```python
from build123d import *

# Parameters (mm, degrees)
SKETCH007_W     = 120
SKETCH007_H     = 120
PAD002_DEPTH    = 100
POCKET005_DEPTH = 100.001
SKETCH009_R     = 1.9
POCKET006_DEPTH = 16
SKETCH010_W     = 3.9
SKETCH010_H     = 62
POCKET007_DEPTH = 114
SKETCH011_R     = 1.9
POCKET008_DEPTH = 16
SKETCH012_R     = 1.9
POCKET009_DEPTH = 120.001
SKETCH013_W     = 106
SKETCH013_H     = 50
POCKET010_DEPTH = 3
SKETCH014_R     = 3
POCKET011_DEPTH = 120.001
SKETCH015_W     = 10
SKETCH015_H     = 10
POCKET012_DEPTH = 3


with BuildPart() as part:
    # Sketch007 → Pad002 (new body)
    with BuildSketch(Plane.XY):
        with Locations((75, 75)):
            Rectangle(SKETCH007_W, SKETCH007_H)
    extrude(amount=PAD002_DEPTH)

    # Sketch008 (on Face5 of Pad002) → Pocket005 (cut, through all)
    with BuildSketch(Plane(origin=(0, 0, 0), x_dir=(1, 0, 0), z_dir=(0, 0, -1))):
        with BuildLine():
            Line((21.9, -18), (128.1, -18))
            Line((128.1, -18), (128.1, -18.9))
            ThreePointArc((128.1, -18.9), (128.97868, -21.02132), (131.1, -21.9))
            Line((132, -21.9), (131.1, -21.9))
            Line((132, -21.9), (132, -128.1))
            Line((132, -128.1), (131.1, -128.1))
            ThreePointArc((131.1, -128.1), (128.97868, -128.97868), (128.1, -131.1))
            Line((128.1, -132), (128.1, -131.1))
            Line((21.9, -132), (128.1, -132))
            Line((21.9, -132), (21.9, -131.1))
            ThreePointArc((21.9, -131.1), (21.02132, -128.97868), (18.9, -128.1))
            Line((18, -128.1), (18.9, -128.1))
            Line((18, -21.9), (18, -128.1))
            Line((18, -21.9), (18.9, -21.9))
            ThreePointArc((18.9, -21.9), (21.02132, -21.02132), (21.9, -18.9))
            Line((21.9, -18), (21.9, -18.9))
        make_face()
    extrude(amount=-POCKET005_DEPTH, mode=Mode.SUBTRACT)

    # Sketch009 (on Face5 of Pocket005) → Pocket006 (cut)
    with BuildSketch(Plane.XY.offset(100)):
        with Locations((18.9, 18.9)):
            Circle(SKETCH009_R)
        with Locations((131.1, 18.9)):
            Circle(SKETCH009_R)
        with Locations((131.1, 131.1)):
            Circle(SKETCH009_R)
        with Locations((18.9, 131.1)):
            Circle(SKETCH009_R)
    extrude(amount=-POCKET006_DEPTH, mode=Mode.SUBTRACT)

    # Sketch010 (on Face7 of Pocket006) → Pocket007 (cut)
    with BuildSketch(Plane.YZ.offset(18)):
        with Locations((19.95, 50)):
            Rectangle(SKETCH010_W, SKETCH010_H)
        with Locations((130.05, 50)):
            Rectangle(SKETCH010_W, SKETCH010_H)
    extrude(amount=POCKET007_DEPTH, mode=Mode.SUBTRACT)

    # Sketch011 (on Face4 of Pocket007) → Pocket008 (cut)
    with BuildSketch(Plane(origin=(0, 0, 0), x_dir=(1, 0, 0), z_dir=(0, 0, -1))):
        with Locations((18.9, -131.1)):
            Circle(SKETCH011_R)
        with Locations((18.9, -18.9)):
            Circle(SKETCH011_R)
        with Locations((131.1, -18.9)):
            Circle(SKETCH011_R)
        with Locations((131.1, -131.1)):
            Circle(SKETCH011_R)
    extrude(amount=-POCKET008_DEPTH, mode=Mode.SUBTRACT)

    # Sketch012 (on Face2 of Pocket008) → Pocket009 (cut, through all)
    with BuildSketch(Plane(origin=(15, 0, 0), x_dir=(0, -1, 0), z_dir=(-1, 0, 0))):
        with Locations((-37.1, 57)):
            Circle(SKETCH012_R)
        with Locations((-37.1, 49.5)):
            Circle(SKETCH012_R)
        with Locations((-93, 57)):
            Circle(SKETCH012_R)
        with Locations((-93, 49.5)):
            Circle(SKETCH012_R)
    extrude(amount=-POCKET009_DEPTH, mode=Mode.SUBTRACT)

    # Sketch013 (on Face6 of Pocket009) → Pocket010 (cut)
    with BuildSketch(Plane.XZ.offset(-15)):
        with Locations((75, 25)):
            Rectangle(SKETCH013_W, SKETCH013_H)
    extrude(amount=-POCKET010_DEPTH, mode=Mode.SUBTRACT)

    # Sketch014 (on Face2 of Pocket010) → Pocket011 (cut, through all)
    with BuildSketch(Plane(origin=(15, 0, 0), x_dir=(0, -1, 0), z_dir=(-1, 0, 0))):
        with Locations((-42.7, 6)):
            Circle(SKETCH014_R)
    extrude(amount=-POCKET011_DEPTH, mode=Mode.SUBTRACT)

    # Sketch015 (on Face1 of Pocket011) → Pocket012 (cut)
    with BuildSketch(Plane(origin=(0, 135, 0), x_dir=(-1, 0, 0), z_dir=(0, 1, 0))):
        with Locations((-123, 15)):
            Rectangle(SKETCH015_W, SKETCH015_H)
    extrude(amount=-POCKET012_DEPTH, mode=Mode.SUBTRACT)


with BuildPart() as part_1:
    # Body009 placement: moved
    add(part.part.moved(Location((0, 0, -44))))


solid = part_1.part
```
Can you work these out from the model? Positions are in its coordinate system, mm. A direction names the side the tool comes from. Give positions to 0.01 mm unless a question says otherwise; leave off trailing zeros. Order: outer loops, then holes, each group sorted by start corner. A loop starts at its lowest first (then second) coordinate and runs counter-clockwise, first axis right, second up. Notation, with made-up numbers: M -11,6.25 L 3,6.25 A21 cw 3,37.25 Z; hole C 7.25,73.5 d6. An arc over 180 degrees is marked long. One line per item, written item: value.
1) I want a section at D-D, the plane z = 13. List the corners of the cut face in (x, y) for me, plus the area to 3 significant figures.
Answer sheet:
outline: M 15,15 L 135,15 L 135,35.2 L 132,35.2 L 132,18 L 18,18 L 18,35.2 L 15,35.2 Z; M 15,39 L 18,39 L 18,91.1 L 15,91.1 Z; M 15,94.9 L 18,94.9 L 18,132 L 132,132 L 132,94.9 L 135,94.9 L 135,135 L 15,135 Z; M 132,39 L 135,39 L 135,91.1 L 132,91.1 Z
area: 1,360 mm^2
2) On a 3-axis mill with a long thin cutter (end or side, diameter ignored), from which of +Z, -Z, +X, -X, +Y, -Y can I reach the whole of each face in a straight line? I mean faces 4 (the face through (22, 16, -19)), 5 (the face through (20, 130, 37)), 6 (the face through (132.912, 131.671, 48.112)), 7 (the face through (129, 128.96, 46.37)), 8 (the face through (131, 131, -28)). Say none if no direction works.
Answer sheet:
face 4: -Z, -Y
face 5: none
face 6: +Z
face 7: +Z, -Z
face 8: -Z
3) Please list where these lines run through material, in increasing order: line 1 along Y through (x, z) = (18.9, 50.75); line 2 along X through (y, z) = (114.5, -17).
Answer sheet:
line 1: y = 15 to 17, 20.8 to 21.9, 128.1 to 129.2, 133 to 135
line 2: x = 15 to 18, 132 to 135
4) I want a section at B-B, the plane x = 37.5. List the corners of the cut face in (y, z) for me.
Answer sheet:
outline: M 15,6 L 18,6 L 18,56 L 15,56 Z; M 132,-44 L 135,-44 L 135,56 L 132,56 Z
5) For P1, Ø1.9, axis at x = 19.5, y = 20, coming from the +Z side; P2, Ø1.9, axis at x = 19.5, y = 131, coming from the -Z side; P3, Ø3, axis at x = 131.1, y = 18.9, coming from the +Z side, each with a flat end and sliding along its axis, tell me the tip position at first contact or that it passes through.
Answer sheet:
P1: stops at z = 56
P2: stops at z = -28
P3: stops at z = 40
6) I want a section at A-A, the plane y = 42.7. List the corners of the cut face in (x, z) for me.
Answer sheet:
outline: M 15,-44 L 18,-44 L 18,-41 L 15,-41 Z; M 15,-35 L 18,-35 L 18,56 L 15,56 Z; M 132,-44 L 135,-44 L 135,-41 L 132,-41 Z; M 132,-35 L 135,-35 L 135,56 L 132,56 Z
7) I want a section at C-C, the plane y = 70. List the corners of the cut face in (x, z) for me, plus the area to 3 significant figures.
Answer sheet:
outline: M 15,-44 L 18,-44 L 18,56 L 15,56 Z; M 132,-44 L 135,-44 L 135,56 L 132,56 Z
area: 600 mm^2
8) We'd pull the mould along Y, two halves only. Please class faces 1 (the face through (74, 15, 28)), 2 (the face through (128, 16, -19)), 3 (the face through (133.48, 39.84, -37.1)): released by +Y, released by -Y, zero draft, split by the parting line, or undercut.
Answer sheet:
face 1: released by -Y
face 2: zero draft
face 3: undercut
